```python
from build123d import *

# Parameters (mm, degrees)
SKETCH1_W           = 106
SKETCH1_H           = 106
BOSS_EXTRUDE1_DEPTH = 10
SKETCH3_W           = 100
SKETCH3_H           = 100
CUT_EXTRUDE5_DEPTH  = 7
CUT_EXTRUDE9_DEPTH  = 1.5
SKETCH14_R          = 1
CUT_EXTRUDE10_DEPTH = 115.5
CUT_EXTRUDE11_START = -1.5
SKETCH15_R          = 1.75
CUT_EXTRUDE11_DEPTH = 1.5
FILLET1_R           = 5


with BuildPart() as part:
    # Sketch1 → Boss-Extrude1 (new body)
    with BuildSketch(Plane(origin=(0, 0, 0), x_dir=(1, 0, 0), z_dir=(0, 1, 0))):
        Rectangle(SKETCH1_W, SKETCH1_H)
    extrude(amount=BOSS_EXTRUDE1_DEPTH)

    # Sketch3 → Cut-Extrude5 (cut)
    with BuildSketch(Plane(origin=(0, 10, 0), x_dir=(1, 0, 0), z_dir=(0, 1, 0))):
        Rectangle(SKETCH3_W, SKETCH3_H)
    extrude(amount=-CUT_EXTRUDE5_DEPTH, mode=Mode.SUBTRACT)

    # Sketch12 → Cut-Extrude9 (cut)
    with BuildSketch(Plane(origin=(53, 0, 0), x_dir=(0, 0, -1), z_dir=(1, 0, 0))):
        with BuildLine():
            ThreePointArc((-17.75, 5), (-18.262563133, 6.237436867), (-19.5, 6.75))
            Line((-19.5, 6.75), (-19.5, 3.25))
            ThreePointArc((-19.5, 3.25), (-18.262563133, 3.762563133), (-17.75, 5))
        make_face()
        with BuildLine():
            Line((-19.5, 3.25), (-19.5, 6.75))
            ThreePointArc((-19.5, 6.75), (-21.25, 5), (-19.5, 3.25))
        make_face()
        with BuildLine():
            ThreePointArc((21.25, 5), (20.737436867, 6.237436867), (19.5, 6.75))
            Line((19.5, 6.75), (19.5, 3.25))
            ThreePointArc((19.5, 3.25), (20.737436867, 3.762563133), (21.25, 5))
        make_face()
        with BuildLine():
            Line((19.5, 3.25), (19.5, 6.75))
            ThreePointArc((19.5, 6.75), (17.75, 5), (19.5, 3.25))
        make_face()
    extrude(amount=-CUT_EXTRUDE9_DEPTH, mode=Mode.SUBTRACT)

    # Sketch14 → Cut-Extrude10 (cut)
    with BuildSketch(Plane(origin=(51.5, 0, 0), x_dir=(0, 0, -1), z_dir=(1, 0, 0))):
        with Locations((-19.5, 5)):
            Circle(SKETCH14_R)
        with Locations((19.5, 5)):
            Circle(SKETCH14_R)
    extrude(amount=-CUT_EXTRUDE10_DEPTH, mode=Mode.SUBTRACT)

    # Sketch15 → Cut-Extrude11 (cut)
    with BuildSketch(Plane.ZY.offset(53).offset(CUT_EXTRUDE11_START)):
        with Locations(Location((-19.5, 5, 0), (0, 0, 180))):
            Circle(SKETCH15_R)
        with Locations(Location((19.5, 5, 0), (0, 0, 180))):
            Circle(SKETCH15_R)
    extrude(amount=CUT_EXTRUDE11_DEPTH, mode=Mode.SUBTRACT)

    # Fillet1
    fillet1_edges = [part.edges().sort_by_distance(p)[0] for p in [
        (53, 5, 53),
        (-53, 5, 53),
        (-53, 5, -53),
        (53, 5, -53),
    ]]
    fillet(fillet1_edges, radius=FILLET1_R)


solid = part.part
```
Design review of the part built by this model. Coordinates are the model's own, in mm. A direction names the side the tool comes from. Give positions to 0.01 mm unless a question says otherwise; leave off trailing zeros. Loops run counter-clockwise (first coordinate to the right, second up) from the corner with the lowest first, then second, coordinate; pieces in that order, holes last. Notation, with made-up numbers: M -4,-35 L 53,-35 A23 cw 53,-5 Z; hole C 69,61 d2. An arc over 180 degrees is marked long. Return JSON: item names as keys, results as strings. Group by question number.
Item 1: Mouldability with a two-part tool opening along Z and no side actions: class faces 1 (the flat face through (50, 7, 1)), 2 (the flat face through (-1, 5, 53)), 3 (the flat face through (-53, 5, 1)), 4 (the flat face through (51.5, 5, -21)) as released by +Z, released by -Z, zero draft, split by the parting line, or undercut.
Item 2: We need section A-A (z = 31). Give the boundary of the cut face in (x, y), and give its area (3 significant figures).
Item 3: Tool access review of faces 5 (the flat face through (-51.5, 5, -21)), 6 (the flat face through (-1, 7, -50)), 7 (the flat face through (51.5, 5, 18)): name each direction out of +Z, -Z, +X, -X, +Y, -Y from which nothing blocks a thin tool from reaching the whole face with its end or side.
Item 4: Insertion check: pin 1 Ø6 at (x, z) = (31, -8.5) entering from +Y; pin 2 Ø2.5 at (y, z) = (5, 19.5) entering from +X; pin 3 Ø2.5 at (y, z) = (5, 19.5) entering from -X; pin 4 Ø1.2 at (y, z) = (5, -19.5) entering from +X. Each pin has a flat end and moves straight along its axis. Give the tip position at first contact, or say it passes through.
Item 5: For probe 1 along Y at (x, z) = (-50.55, 19.5); probe 2 along Z at (x, y) = (-5.5, 9.25), list the stretches that pass through material, from the lowest coordinate up.
Item 6: We need section B-B (x = -44.5). Give the boundary of the cut face in (y, z), and give its area (3 significant figures).
Output:
{
 "1": {"face 1": "undercut", "face 2": "released by +Z", "face 3": "zero draft", "face 4": "undercut"},
 "2": {"outline": "M -53,0 L 53,0 L 53,10 L 50,10 L 50,3 L -50,3 L -50,10 L -53,10 Z", "area": "360 mm^2"},
 "3": {"face 5": "-X", "face 6": "+Y", "face 7": "+X"},
 "4": {"pin 1": "stops at y = 3", "pin 2": "stops at x = 51.5", "pin 3": "stops at x = -51.5", "pin 4": "passes through"},
 "5": {"probe 1": "y = 0 to 4, 6 to 10", "probe 2": "z = -53 to -50, 50 to 53"},
 "6": {"outline": "M 0,-53 L 10,-53 L 10,-50 L 3,-50 L 3,50 L 10,50 L 10,53 L 0,53 Z", "area": "360 mm^2"}
}
